```python
from build123d import *

# Parameters (mm, degrees)
BOSS_EXTRUDE1_DEPTH     = 3
SKETCH4_W               = 5
SKETCH4_H               = 20
BOSS_EXTRUDE2_DEPTH     = 25
FILLET3_R               = 10
CUT_EXTRUDE3_DEPTH      = 121.479251326
CUT_EXTRUDE3_DEPTH_BACK = 121.479251326
SKETCH5_R               = 2.75
CUT_EXTRUDE4_DEPTH      = 2.5
CHAMFER1_SIZE           = 5
CHAMFER3_SIZE           = 2.5
SKETCH7_W               = 30
SKETCH7_H               = 3
BOSS_EXTRUDE3_DEPTH     = 50
CHAMFER4_SIZE           = 10


with BuildPart() as part:
    # Sketch1 → Boss-Extrude1 (new body)
    with BuildSketch(Plane(origin=(0, 0, 0), x_dir=(1, 0, 0), z_dir=(0, 1, 0))):
        with BuildLine():
            Line((-10, 15), (10, 15))
            ThreePointArc((10, 15), (45.355339059, 29.644660941), (60, 65))
            Line((60, 65), (90, 65))
            ThreePointArc((90, 65), (66.568542495, 8.431457505), (10, -15))
            Line((10, -15), (-10, -15))
            ThreePointArc((-10, -15), (-66.568542495, 8.431457505), (-90, 65))
            Line((-90, 65), (-60, 65))
            ThreePointArc((-60, 65), (-45.355339059, 29.644660941), (-10, 15))
        make_face()
    extrude(amount=BOSS_EXTRUDE1_DEPTH)

    # Sketch4 → Boss-Extrude2 (add)
    with BuildSketch(Plane(origin=(0, 3, 0), x_dir=(1, 0, 0), z_dir=(0, 1, 0))):
        with Locations((-5, 0)):
            Rectangle(SKETCH4_W, SKETCH4_H)
        with Locations((5, 0)):
            Rectangle(SKETCH4_W, SKETCH4_H)
    extrude(amount=BOSS_EXTRUDE2_DEPTH)

    # Fillet3
    fillet3_edges = [part.edges().sort_by_distance(p)[0] for p in [
        (5, 28, 10),
        (5, 28, -10),
        (-5, 28, -10),
        (-5, 28, 10),
    ]]
    fillet(fillet3_edges, radius=FILLET3_R - 0.0001)  # a hair under: the kernel refuses the full size

    # Sketch5 → Cut-Extrude3 (cut, two sides: drawn at the far end of the back side and taken through both)
    with BuildSketch(Plane.ZY.offset(7.5).offset(-CUT_EXTRUDE3_DEPTH_BACK)):
        with Locations((0, 18)):
            Circle(SKETCH5_R)
    extrude(amount=CUT_EXTRUDE3_DEPTH + CUT_EXTRUDE3_DEPTH_BACK, mode=Mode.SUBTRACT)

    # Sketch6 → Cut-Extrude4 (cut)
    with BuildSketch(Plane(origin=(7.5, 0, 0), x_dir=(0, 0, -1), z_dir=(1, 0, 0))):
        Polygon((0, 13.236860279), (4.125, 15.61843014), (4.125, 20.38156986), (0, 22.763139721), (-4.125, 20.38156986), (-4.125, 15.61843014), align=None)
    extrude(amount=-CUT_EXTRUDE4_DEPTH, mode=Mode.SUBTRACT)

    # Chamfer1
    chamfer1_edges = [part.edges().sort_by_distance(p)[0] for p in [
        (-5, 3, -10),
        (-5, 3, 10),
        (5, 3, -10),
        (5, 3, 10),
    ]]
    chamfer(chamfer1_edges, length=CHAMFER1_SIZE - 0.0001)  # a hair under: the kernel refuses the full size

    # Chamfer3
    chamfer3_edges = [part.edges().sort_by_distance(p)[0] for p in [
        (-2.5, 3, 0),
        (-7.5, 3, 0),
        (2.5, 3, 0),
        (7.5, 3, 0),
    ]]
    chamfer(chamfer3_edges, length=CHAMFER3_SIZE - 0.0001)  # a hair under: the kernel refuses the full size

    # Sketch7 → Boss-Extrude3 (add)
    with BuildSketch(Plane(origin=(0, 0, -65), x_dir=(-1, 0, 0), z_dir=(0, 0, -1))):
        with Locations((-75, 1.5)):
            Rectangle(SKETCH7_W, SKETCH7_H)
        with Locations((75, 1.5)):
            Rectangle(SKETCH7_W, SKETCH7_H)
    extrude(amount=BOSS_EXTRUDE3_DEPTH)

    # Chamfer4
    chamfer4_edges = [part.edges().sort_by_distance(p)[0] for p in [
        (90, 1.5, -115),
        (60, 1.5, -115),
        (-60, 1.5, -115),
        (-90, 1.5, -115),
    ]]
    chamfer(chamfer4_edges, length=CHAMFER4_SIZE)


solid = part.part
```
Input: part model. Units: mm. Frame: model coordinates. A direction names the side the tool comes from. Coordinates: 2 decimals unless noted, no trailing zeros. Loops run counter-clockwise (first coordinate to the right, second up) from the corner with the lowest first, then second, coordinate; pieces in that order, holes last. Notation, with made-up numbers: (64, 42) - (98, 42) arc R15 cw to (98, 61) - close; hole circle Ø11 at (50, 9.5). An arc over 180 degrees is marked (long way). Answer in a Markdown table with one row per item.
(1) Set-up query: faces 4 (the face through (65, 1, -110)), 5 (the face through (2.5, 14, 0)), 6 (the face through (5, 13, 10)), 7 (the face through (-7.5, 14, 0)). Return all of +Z, -Z, +X, -X, +Y, -Y with unobstructed straight access to the full face (end or side cutting, diameter ignored); none if empty.
Model answer:
| item | result |
|---|---|
| face 4 | -Z, +Y, -Y |
| face 5 | +Z, -Z, +Y |
| face 6 | +Z, +X, -X, +Y |
| face 7 | +Z, -Z, -X, +Y |
(2) Mould query, pull axis Y, two halves, no side actions, for faces 1 (the face through (-4.96, 24.99, -7.15)), 2 (the face through (5, 18, 3)), 3 (the face through (85, 1, -110)). Classes: pulls with the +Y half, pulls with the -Y half, needs draft (parallel to the pull), parting line crosses it, or undercut.
Model answer:
| item | result |
|---|---|
| face 1 | pulls with the +Y half |
| face 2 | undercut |
| face 3 | needs draft |
(3) Cut plane A-A on z = -82. Output: boundary loops of the cut face in (x, y), plus the area to 3 significant figures.
Model answer:
| item | result |
|---|---|
| outline | (-90, 0) - (-60, 0) - (-60, 3) - (-90, 3) - close; (60, 0) - (90, 0) - (90, 3) - (60, 3) - close |
| area | 180 mm² |
(4) Material intervals for L1, parallel to Z at x = -6.3, y = 18; L2, parallel to Y at x = -6.2, z = 0; L3, parallel to X at y = 21.25, z = -6, sorted ascending. Write a range as from..to.
Model answer:
| item | result |
|---|---|
| L1 | z = -10..-2.75, 2.75..10 |
| L2 | y = 0..15.25, 20.75..28 |
| L3 | x = -7.5..-2.5, 2.5..7.5 |
(5) Pin query (flat end, axial travel): P1, Ø1.5, axis at x = 4.5, y = 14, coming from the +Z side; P2, Ø5.5, axis at x = -4.5, y = 14, coming from the -Z side; P3, Ø9, axis at y = 18, z = 0, coming from the +X side. Return the tip coordinate at first contact, or that it passes through.
Model answer:
| item | result |
|---|---|
| P1 | stops at z = 10 |
| P2 | stops at z = -10 |
| P3 | stops at x = 7.5 |
